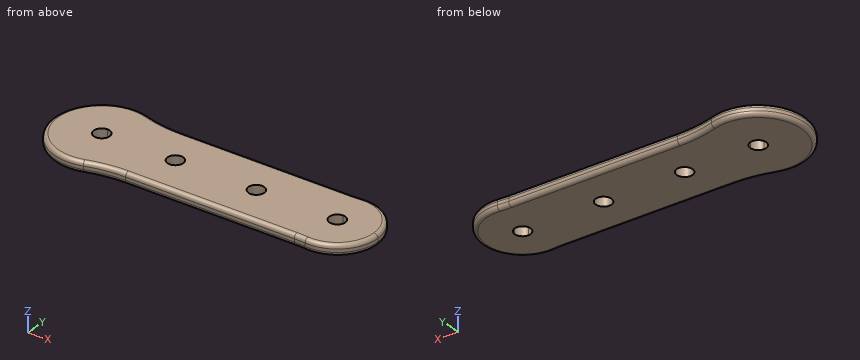
```python
from build123d import *

# Parameters (mm, degrees)
SKETCH1_R           = 5
BOSS_EXTRUDE1_DEPTH = 7
FILLET1_R           = 80
FILLET2_R           = 2.5


with BuildPart() as part:
    # Sketch1 → Boss-Extrude1 (new body)
    # profile 1 of 9: a face of its own
    with BuildSketch(Plane.XY):
        with BuildLine():
            Line((69.410011136, 25), (-57.316876048, 25))
            ThreePointArc((-57.316876048, 25), (-47.466179631, 14.186371655), (-43.9, 0))
            ThreePointArc((-43.9, 0), (-47.466179631, -14.186371655), (-57.316876048, -25))
            Line((-57.316876048, -25), (69.410011136, -25))
            ThreePointArc((69.410011136, -25), (48.5, 0), (69.410011136, 25))
        make_face()
        with Locations((-27.7, 0)):
            Circle(SKETCH1_R, mode=Mode.SUBTRACT)
        with Locations((23.1, 0)):
            Circle(SKETCH1_R, mode=Mode.SUBTRACT)
    # profile 2 of 9: a face of its own
    with BuildSketch(Plane.XY):
        with BuildLine():
            ThreePointArc((99.3, 0), (90.195924074, 19.483399564), (69.410011136, 25))
            Line((69.410011136, 25), (73.9, 25))
            Line((73.9, 25), (73.9, 5))
            ThreePointArc((73.9, 5), (77.435533906, 3.535533906), (78.9, 0))
            ThreePointArc((78.9, 0), (77.435533906, -3.535533906), (73.9, -5))
            Line((73.9, -5), (73.9, -25))
            Line((73.9, -25), (69.410011136, -25))
            ThreePointArc((69.410011136, -25), (90.195924074, -19.483399564), (99.3, 0))
        make_face()
    # profile 3 of 9: a face of its own
    with BuildSketch(Plane.XY):
        with BuildLine():
            Line((73.9, 25), (69.410011136, 25))
            ThreePointArc((69.410011136, 25), (48.5, 0), (69.410011136, -25))
            Line((69.410011136, -25), (73.9, -25))
            Line((73.9, -25), (73.9, -5))
            ThreePointArc((73.9, -5), (68.9, 0), (73.9, 5))
            Line((73.9, 5), (73.9, 25))
        make_face()
    # profile 4 of 9: a face of its own
    with BuildSketch(Plane.XY):
        with BuildLine():
            ThreePointArc((99.3, 0), (90.195924074, 19.483399564), (69.410011136, 25))
            Line((69.410011136, 25), (73.9, 25))
            Line((73.9, 25), (73.9, 5))
            ThreePointArc((73.9, 5), (77.435533906, 3.535533906), (78.9, 0))
            ThreePointArc((78.9, 0), (77.435533906, -3.535533906), (73.9, -5))
            Line((73.9, -5), (73.9, -25))
            Line((73.9, -25), (69.410011136, -25))
            ThreePointArc((69.410011136, -25), (90.195924074, -19.483399564), (99.3, 0))
        make_face()
    # profile 5 of 9: a face of its own
    with BuildSketch(Plane.XY):
        with BuildLine():
            Line((73.9, 25), (69.410011136, 25))
            ThreePointArc((69.410011136, 25), (48.5, 0), (69.410011136, -25))
            Line((69.410011136, -25), (73.9, -25))
            Line((73.9, -25), (73.9, -5))
            ThreePointArc((73.9, -5), (68.9, 0), (73.9, 5))
            Line((73.9, 5), (73.9, 25))
        make_face()
    # profile 6 of 9: a face of its own
    with BuildSketch(Plane.XY):
        with BuildLine():
            Line((-73.9, 5), (-73.9, 25))
            Line((-73.9, 25), (-57.316876048, 25))
            ThreePointArc((-57.316876048, 25), (-103.9, 0), (-57.316876048, -25))
            Line((-57.316876048, -25), (-73.9, -25))
            Line((-73.9, -25), (-73.9, -5))
            ThreePointArc((-73.9, -5), (-78.9, 0), (-73.9, 5))
        make_face()
    # profile 7 of 9: a face of its own
    with BuildSketch(Plane.XY):
        with BuildLine():
            Line((-57.316876048, 25), (-73.9, 25))
            Line((-73.9, 25), (-73.9, 5))
            ThreePointArc((-73.9, 5), (-70.364466094, 3.535533906), (-68.9, 0))
            ThreePointArc((-68.9, 0), (-70.364466094, -3.535533906), (-73.9, -5))
            Line((-73.9, -5), (-73.9, -25))
            Line((-73.9, -25), (-57.316876048, -25))
            ThreePointArc((-57.316876048, -25), (-47.466179631, -14.186371655), (-43.9, 0))
            ThreePointArc((-43.9, 0), (-47.466179631, 14.186371655), (-57.316876048, 25))
        make_face()
    # profile 8 of 9: a face of its own
    with BuildSketch(Plane.XY):
        with BuildLine():
            Line((-73.9, 5), (-73.9, 25))
            Line((-73.9, 25), (-57.316876048, 25))
            ThreePointArc((-57.316876048, 25), (-103.9, 0), (-57.316876048, -25))
            Line((-57.316876048, -25), (-73.9, -25))
            Line((-73.9, -25), (-73.9, -5))
            ThreePointArc((-73.9, -5), (-78.9, 0), (-73.9, 5))
        make_face()
    # profile 9 of 9: a face of its own
    with BuildSketch(Plane.XY):
        with BuildLine():
            Line((-57.316876048, 25), (-73.9, 25))
            Line((-73.9, 25), (-73.9, 5))
            ThreePointArc((-73.9, 5), (-70.364466094, 3.535533906), (-68.9, 0))
            ThreePointArc((-68.9, 0), (-70.364466094, -3.535533906), (-73.9, -5))
            Line((-73.9, -5), (-73.9, -25))
            Line((-73.9, -25), (-57.316876048, -25))
            ThreePointArc((-57.316876048, -25), (-47.466179631, -14.186371655), (-43.9, 0))
            ThreePointArc((-43.9, 0), (-47.466179631, 14.186371655), (-57.316876048, 25))
        make_face()
    extrude(amount=BOSS_EXTRUDE1_DEPTH)

    # Fillet1
    fillet1_edges = [part.edges().sort_by_distance(p)[0] for p in [
        (-57.316876048, 25, 3.5),
        (69.410011136, 25, 3.5),
        (69.410011136, -25, 3.5),
        (-57.316876048, -25, 3.5),
    ]]
    fillet(fillet1_edges, radius=FILLET1_R)

    # Fillet2
    fillet2_edges = [part.edges().sort_by_distance(p)[0] for p in [
        (99.3, 0, 0),
        (99.3, 0, 7),
        (11.806658334, -25, 0),
        (11.806658334, -25, 7),
        (11.806658334, 25, 0),
        (11.806658334, 25, 7),
        (-103.9, 0, 0),
        (-103.9, 0, 7),
        (68.210978782, -25.075937369, 0),
        (68.210978782, -25.075937369, 7),
        (68.210978782, 25.075937369, 0),
        (68.210978782, 25.075937369, 7),
        (-53.173261162, -25.914315742, 0),
        (-53.173261162, -25.914315742, 7),
        (-53.173261162, 25.914315742, 0),
        (-53.173261162, 25.914315742, 7),
    ]]
    fillet(fillet2_edges, radius=FILLET2_R)


solid = part.part
```
Read the model definition and answer for the solid it produces. Units are mm, in the model's axes. Give positions to 0.01 mm unless a question says otherwise; leave off trailing zeros. Loops run counter-clockwise (first coordinate to the right, second up) from the corner with the lowest first, then second, coordinate; pieces in that order, holes last.
Item 1: Each of these flat-tipped pins is pushed along its axis until it touches: pin 1 Ø1 at (x, z) = (37, 4) entering from +Y; pin 2 Ø1 at (x, z) = (-18.5, 2) entering from -Y; pin 3 Ø2 at (x, z) = (27, 1) entering from +Y. Where does it stop, or does it pass through?
Item 2: The part is cut by section B-B (y = 3). Give the number of separate pieces and of enclosed holes in the cut face, and give its area (3 significant figures).
Item 3: The part is cut by section A-A (x = 23.1). Write down the section's boundary in (y, z).
Item 4: Find the intervals of material crossed by line 1 along Y through (x, z) = (23.1, 3); line 2 along X through (y, z) = (-2, 0.5); line 3 along Y through (x, z) = (63, 3), in increasing order.
Taken from the geometry:
1. pin 1: stops at y = 25
1. pin 2: stops at y = -25
1. pin 3: stops at y = 24.95
2. separate pieces: 5
2. enclosed holes: 0
2. area: 1,190 mm2
3. outline: (-25, 2.5) arc R2.5 ccw to (-22.5, 0) - (-5, 0) - (-5, 7) - (-22.5, 7) arc R2.5 ccw to (-25, 4.5) - close; (5, 0) - (22.5, 0) arc R2.5 ccw to (25, 2.5) - (25, 4.5) arc R2.5 ccw to (22.5, 7) - (5, 7) - close
4. line 1: y = -25 to -5, 5 to 25
4. line 2: x = -102.83 to -78.48, -69.32 to -32.28, -23.12 to 18.52, 27.68 to 69.32, 78.48 to 98.22
4. line 3: y = -25 to 25
